from build123d import *

# Parameters (mm, degrees)
SKETCH1_R             = 22.5
BOSS_EXTRUDE2_DEPTH   = 20
F_4_0MM_DOWEL_HOLE1_D = 4


with BuildPart() as part:
    # Sketch1 → Boss-Extrude2 (new body)
    with BuildSketch(Plane.XY.offset(-167.5)):
        with BuildLine():
            Line((-32.5, 0), (-32.5, -15))
            Line((-32.5, -15), (-52.5, -15))
            Line((-52.5, -15), (-52.5, -25))
            Line((-52.5, -25), (52.5, -25))
            Line((52.5, -25), (52.5, -15))
            Line((52.5, -15), (32.5, -15))
            Line((32.5, -15), (32.5, 0))
            ThreePointArc((32.5, 0), (0, 32.5), (-32.5, 0))
        make_face()
        Circle(SKETCH1_R, mode=Mode.SUBTRACT)
    extrude(amount=-BOSS_EXTRUDE2_DEPTH)

    # Ø4.0mm Dowel Hole1 (through all)
    with Locations(Plane(origin=(0, -15, 0), x_dir=(1, 0, 0), z_dir=(0, 1, 0))):
        with Locations((42.5, 177.5), (-42.5, 177.5)):
            Hole(F_4_0MM_DOWEL_HOLE1_D / 2)


solid = part.part
CAD build for the part. Positions are in the model's coordinates, mm. A direction names the side the tool comes from. Give positions to 0.01 mm unless a question says otherwise; leave off trailing zeros. Write each loop counter-clockwise with the first axis right and the second up, starting at its lowest first coordinate (ties: lowest second). Pieces come first, ordered by that corner, then holes. Notation, with made-up numbers: (63.25, -7.75) - (121.25, -7.75) arc R31 cw to (121.25, 24.25) - close; hole circle Ø1 at (-5.5, 4.25). An arc over 180 degrees is marked (long way). Put each result on its own line as item: value.
(1) Pull direction Z, two halves, no side cores. Call faces 1 (the flat face through (23, -2, -167.5)), 2 (the flat face through (32.5, -8, -177)), 3 (the cylindrical face through (-43.423, -20.07, -175.726)): released by +Z, released by -Z, zero draft, split by the parting line, or undercut.
Working result:
face 1: released by +Z
face 2: zero draft
face 3: undercut
(2) Saw through at C-C (y = -2). List the corners of the cut face in (x, z), then the cut area to 3 significant figures.
Working result:
outline: (-32.5, -187.5) - (-22.41, -187.5) - (-22.41, -167.5) - (-32.5, -167.5) - close; (22.41, -187.5) - (32.5, -187.5) - (32.5, -167.5) - (22.41, -167.5) - close
area: 404 mm^2
(3) Saw through at B-B (z = -171.25). List the corners of the cut face in (x, y), then the cut area to 3 significant figures.
Working result:
outline: (-52.5, -25) - (52.5, -25) - (52.5, -15) - (32.5, -15) - (32.5, 0) arc R32.5 ccw to (-32.5, 0) - (-32.5, -15) - (-52.5, -15) - close; hole circle Ø45 at (0, 0)
area: 2,090 mm^2
(4) Saw through at A-A (x = 0). List the corners of the cut face in (y, z).
Working result:
outline: (-25, -187.5) - (-22.5, -187.5) - (-22.5, -167.5) - (-25, -167.5) - close; (22.5, -187.5) - (32.5, -187.5) - (32.5, -167.5) - (22.5, -167.5) - close
(5) Wall check: L1, parallel to X at y = 0.5, z = -178.5; L2, parallel to Z at x = -42.5, y = -20; L3, parallel to Y at x = 0, z = -173.5. Give the ranges that are in metal, low to high.
Working result:
L1: -32.5 to -22.49, 22.49 to 32.5
L2: -187.5 to -179.5, -175.5 to -167.5
L3: -25 to -22.5, 22.5 to 32.5
(6) Saw through at D-D (y = 28). List the corners of the cut face in (x, z), then the cut area to 3 significant figures.
Working result:
outline: (-16.5, -187.5) - (16.5, -187.5) - (16.5, -167.5) - (-16.5, -167.5) - close
area: 660 mm^2
(7) Tool access for faces 4 (the flat face through (43, -15, -175)), 5 (the cylindrical face through (0.715, 32.492, -177.36)), 6 (the flat face through (-32.5, -7, -177)): list every direction of +Z, -Z, +X, -X, +Y, -Y with a clear straight run to the whole face (end or side of a thin tool).
Working result:
face 4: +Z, -Z, +X, +Y
face 5: +Z, -Z, +Y
face 6: +Z, -Z, -X, +Y
(8) Drop flat-ended pins along their axis: pin 1 Ø1.5 at (x, z) = (-7, -180.5) entering from +Y; pin 2 Ø1 at (x, y) = (14, -15.5) entering from -Z; pin 3 Ø6 at (y, z) = (0.5, -183) entering from +X; pin 4 Ø12 at (y, z) = (-8.5, -179.5) entering from -X. Give the stop position or say it passes through.
Working result:
pin 1: y = 31.89
pin 2: through
pin 3: x = 32.5
pin 4: x = -32.5
